Part model, mm, in its own coordinate system. Face numbers are marked on the shaded views. Coordinates: 2 decimals unless noted, no trailing zeros. Loops run counter-clockwise (first coordinate to the right, second up) from the corner with the lowest first, then second, coordinate; pieces in that order, holes last. Notation, with made-up numbers: M 41.5,55 L 99.5,55 A29 ccw 99.5,76 Z; hole C 39.25,-9.75 d4. An arc over 180 degrees is marked long. Use a Markdown table: item, result. Add a question column.
1) Pin check, flat tip, straight feed: pin 1 Ø6 at (x, y) = (109, 99) entering from -Z. Stop position of the tip, or through.
2) Band-saw the part on B-B (y = 110.5). List the corners of the cut face in (x, z).
3) Band-saw the part on D-D (x = 109). List the corners of the cut face in (y, z).
4) Band-saw the part on A-A (z = 2.9). List the corners of the cut face in (x, y), plus the area to 3 significant figures.
5) Band-saw the part on C-C (x = 134.5). List the corners of the cut face in (y, z).
6) Pull direction Z, two halves, no side cores. Call the marked faces 1, 2, 3 and 4: released by +Z, released by -Z, zero draft, split by the parting line, or undercut.
7) Wall check: probe 1 along Y at (x, z) = (118, 4.1); probe 2 along X at (y, z) = (96, 3.15); probe 3 along Y at (x, z) = (134, 0.25). Give the ranges that are in metal, low to high. Write a range as from..to.
from build123d import *

# Parameters (mm, degrees)
MODEL_R                 = 11
MODEL_R_2               = 1.5
SALIENTE_EXTRUIR1_DEPTH = 5
CROQUIS2_R              = 1.5
CORTAR_EXTRUIR1_DEPTH   = 35


with BuildPart() as part:
    # Model → Saliente-Extruir1 (new body)
    with BuildSketch(Plane.XY):
        with BuildLine():
            Line((112.251450395, 91.173573784), (133.951450395, 91.173573784))
            Line((133.951450395, 91.173573784), (139.601450395, 91.173573784))
            Line((139.601450395, 91.173573784), (139.601450395, 122.873573784))
            Line((139.601450395, 122.873573784), (133.951450395, 122.873573784))
            Line((133.951450395, 122.873573784), (112.251450395, 122.873573784))
            ThreePointArc((112.251450395, 122.873573784), (108.424616072, 122.112369109), (105.180382583, 119.944641596))
            Line((105.180382583, 119.944641596), (105.180382583, 94.102505972))
            ThreePointArc((105.180382583, 94.102505972), (108.424616072, 91.934778459), (112.251450395, 91.173573784))
        make_face()
        with Locations((118.101450395, 107.023573784)):
            Circle(MODEL_R, mode=Mode.SUBTRACT)
        with Locations((135.101450395, 106.173573784)):
            Circle(MODEL_R_2, mode=Mode.SUBTRACT)
        with Locations((135.101450395, 96.173573784)):
            Circle(MODEL_R_2, mode=Mode.SUBTRACT)
    extrude(amount=SALIENTE_EXTRUIR1_DEPTH)

    # Croquis2 → Cortar-Extruir1 (cut)
    with BuildSketch(Plane.XZ.offset(-91.173573784)):
        with Locations(Location((118.101450395, 2.5, 0), (0, 0, 270))):
            Circle(CROQUIS2_R)
    extrude(amount=-CORTAR_EXTRUIR1_DEPTH, mode=Mode.SUBTRACT)


solid = part.part
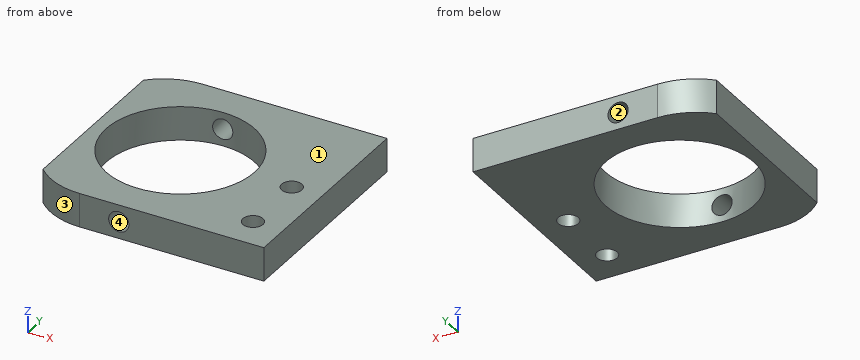
Entries:
| question | item | result |
|---|---|---|
| 1 | pin 1 | z = 0 |
| 2 | outline | M 105.18,0 L 107.67,0 L 107.67,5 L 105.18,5 Z; M 128.54,0 L 139.6,0 L 139.6,5 L 128.54,5 Z |
| 3 | outline | M 91.72,0 L 100.85,0 L 100.85,5 L 91.72,5 Z; M 113.2,0 L 122.33,0 L 122.33,5 L 113.2,5 Z |
| 4 | outline | M 105.18,94.1 A10 ccw 112.25,91.17 L 116.66,91.17 L 116.66,96.12 A11 cw 116.66,117.93 L 116.66,122.87 L 112.25,122.87 A10 ccw 105.18,119.94 Z; M 119.55,91.17 L 139.6,91.17 L 139.6,122.87 L 119.55,122.87 L 119.55,117.93 A11 cw 119.55,96.12 Z; hole C 135.1,96.17 d3; hole C 135.1,106.17 d3 |
| 4 | area | 656 mm2 |
| 5 | outline | M 91.17,0 L 94.8,0 L 94.8,5 L 91.17,5 Z; M 97.55,0 L 104.8,0 L 104.8,5 L 97.55,5 Z; M 107.55,0 L 122.87,0 L 122.87,5 L 107.55,5 Z |
| 6 | face 1 | released by +Z |
| 6 | face 2 | undercut |
| 6 | face 3 | zero draft |
| 6 | face 4 | undercut |
| 7 | probe 1 | 91.17..96.02, 118.02..122.87 |
| 7 | probe 2 | 105.18..116.75, 119.45..133.61, 136.59..139.6 |
| 7 | probe 3 | 91.17..95.16, 97.19..105.16, 107.19..122.87 |
